Could you check a few things on this drawing? It's one solid part, dimensions in mm from its lowest x, y, z. A direction names the side the tool comes from. Give positions to 0.01 mm unless a question says otherwise; leave off trailing zeros. Order: outer loops, then holes, each group sorted by start corner. A loop starts at its lowest first (then second) coordinate and runs counter-clockwise, first axis right, second up. Notation, with made-up numbers: (-11.75, 0.25) -> (19.25, 0.25) arc R19 ccw to (19.25, 18.25) -> close; hole circle Ø10 at (60, 5). An arc over 180 degrees is marked (long way). Answer as CSV lines item,"result".
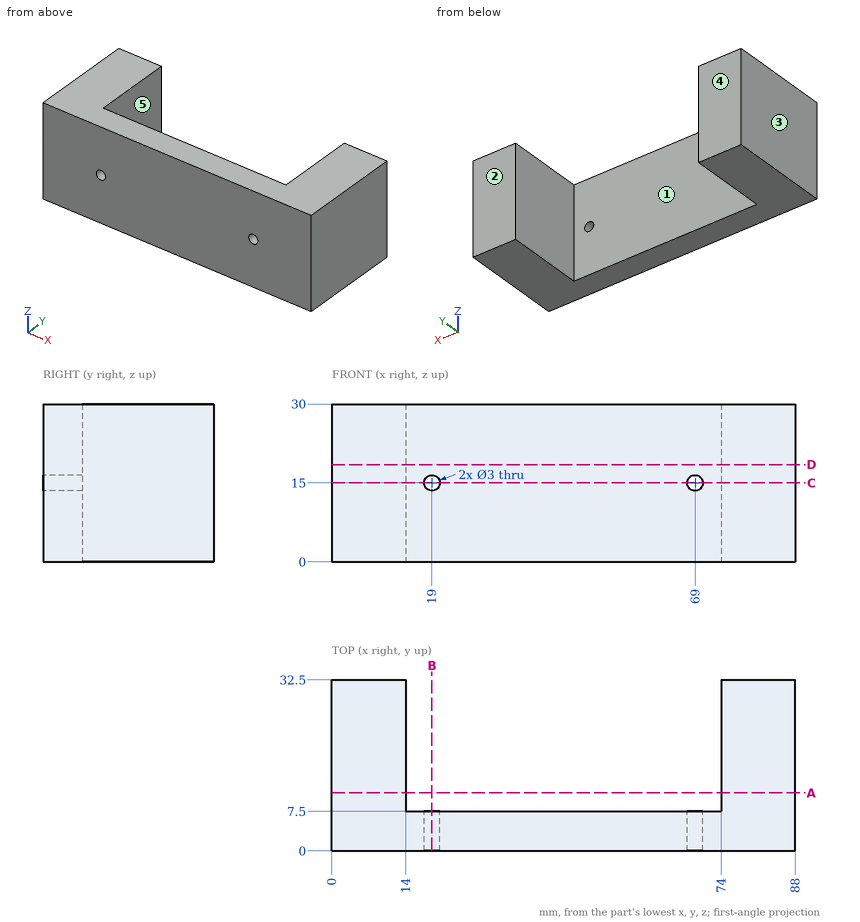
Item 1: Please list where these lines run through material, in increasing order: line 1 along X through (y, z) = (6.25, 15); line 2 along X through (y, z) = (17, 17.5); line 3 along Z through (x, y) = (69, 5.5).
Numbers:
line 1,"x = 0 to 17.5, 20.5 to 67.5, 70.5 to 88"
line 2,"x = 0 to 14, 74 to 88"
line 3,"z = 0 to 13.5, 16.5 to 30"
Item 2: For the marked faces 4 and 5, which set-ups out of +Z, -Z, +X, -X, +Y, -Y let a thin tool reach every point of the face, with its end or its side?
Numbers:
face 4,"+Z, -Z, +X, -X, +Y"
face 5,"+Z, -Z, +Y"
Item 3: Imagine slicing it at A-A, the plane y = 11. Please give me the cut outline in (x, z).
Numbers:
outline,"(0, 0) -> (14, 0) -> (14, 30) -> (0, 30) -> close; (74, 0) -> (88, 0) -> (88, 30) -> (74, 30) -> close"
Item 4: Imagine slicing it at B-B, the plane x = 19. Please give me the cut outline in (y, z).
Numbers:
outline,"(0, 0) -> (7.5, 0) -> (7.5, 13.5) -> (0, 13.5) -> close; (0, 16.5) -> (7.5, 16.5) -> (7.5, 30) -> (0, 30) -> close"
Item 5: Imagine slicing it at D-D, the plane z = 18.5. Please give me the cut outline in (x, y).
Numbers:
outline,"(0, 0) -> (88, 0) -> (88, 32.5) -> (74, 32.5) -> (74, 7.5) -> (14, 7.5) -> (14, 32.5) -> (0, 32.5) -> close"
Item 6: Imagine slicing it at C-C, the plane z = 15. Please give me the cut outline in (x, y), then the cut area to 4 significant figures.
Numbers:
outline,"(0, 0) -> (17.5, 0) -> (17.5, 7.5) -> (14, 7.5) -> (14, 32.5) -> (0, 32.5) -> close; (20.5, 0) -> (67.5, 0) -> (67.5, 7.5) -> (20.5, 7.5) -> close; (70.5, 0) -> (88, 0) -> (88, 32.5) -> (74, 32.5) -> (74, 7.5) -> (70.5, 7.5) -> close"
area,"1,315 mm²"
Item 7: For pin 1 (4 mm diameter, centred on x = 46, z = 15.5, fed in from -Y); pin 2 (12 mm diameter, centred on x = 67, z = 26.5, fed in from +Y), each with a flat end and sliding along its axis, tell me the tip position at first contact or that it passes through.
Numbers:
pin 1,"stops at y = 0"
pin 2,"stops at y = 7.5"
Item 8: We'd pull the mould along X, two halves only. Please class the marked faces 1, 2 and 3: released by +X, released by -X, zero draft, split by the parting line, or undercut.
Numbers:
face 1,"undercut"
face 2,"zero draft"
face 3,"released by -X"
